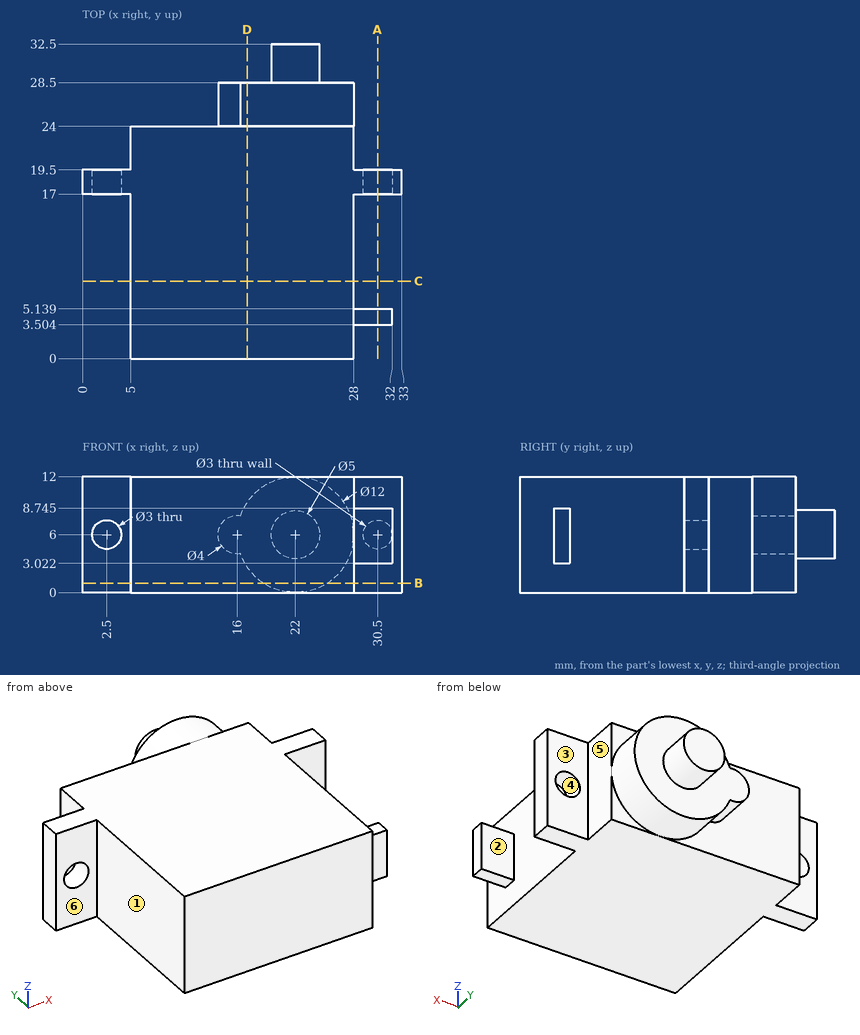
Answer from the drawing. Dimensions are ordinates in mm from the lowest x, y and z of the part. A direction names the side the tool comes from. Coordinates: 2 decimals unless noted, no trailing zeros. Write each loop counter-clockwise with the first axis right and the second up, starting at its lowest first coordinate (ties: lowest second). Pieces come first, ordered by that corner, then holes. Notation, with made-up numbers: M -36.75,76.5 L -28.75,76.5 A7 cw -28.75,85.5 Z; hole C -30,16.25 d11. An arc over 180 degrees is marked long. Put each result on its own line as item: value. Start each with the question number.
1. Which of the six approach directions +Z, -Z, +X, -X, +Y, -Y give full straight-line access (tool end or side, diameter ignored) to the marked faces 1, 2 and 3?
2. A cutting plane is placed at B-B on z = 1. Write down the section's boundary in (x, y).
3. A cutting plane is placed at C-C on y = 8. Write down the section's boundary in (x, z).
4. Flat-ended cylindrical pins translate along their axes: P1, Ø2.5, axis at x = 3, z = 6, coming from the +Y side; P2, Ø2, axis at y = 4.5, z = 2, coming from the -X side; P3, Ø1.8, axis at x = 29.5, y = 4.5, coming from the +Z side (1 decimal). Find the tip coordinate at first contact, or state that the pin passes through.
5. For a pull along X with two mould halves and no side action, classify the marked faces 4, 5 and 6 as pulls with the +X half, pulls with the -X half, needs draft (parallel to the pull), parting line crosses it, or undercut.
6. A cutting plane is placed at A-A on x = 30.5. Write down the section's boundary in (y, z) (1 decimal).
7. A cutting plane is placed at D-D on x = 17. Write down the section's boundary in (y, z).
8. Consider line 1 (X direction, y = 19.05, z = 6); line 2 (Y direction, x = 30.5, z = 4) (1 decimal); line 3 (Z direction, x = 2.5, y = 17.9). Determine where each line is inside the solid, lowest interval first. Write a range as from..to.
Resolved:
1. face 1: +Z, -Z, -X, -Y
1. face 2: +Z, -Z, +X
1. face 3: +Z, -Z, +X, +Y
2. outline: M 0,17 L 5,17 L 5,0 L 28,0 L 28,17 L 33,17 L 33,19.5 L 28,19.5 L 28,24 L 25.32,24 L 25.32,28.5 L 18.68,28.5 L 18.68,24 L 5,24 L 5,19.5 L 0,19.5 Z
3. outline: M 5,0 L 28,0 L 28,12 L 5,12 Z
4. P1: stops at y = 19.5
4. P2: stops at x = 5
4. P3: stops at z = 8.7
5. face 4: undercut
5. face 5: pulls with the +X half
5. face 6: needs draft
6. outline: M 3.5,3 L 5.1,3 L 5.1,8.7 L 3.5,8.7 Z; M 17,0 L 19.5,0 L 19.5,4.5 L 17,4.5 Z; M 17,7.5 L 19.5,7.5 L 19.5,12 L 17,12 Z
7. outline: M 0,0 L 24,0 L 24,2.68 L 28.5,2.68 L 28.5,9.32 L 24,9.32 L 24,12 L 0,12 Z
8. line 1: x = 0..1, 4..29, 32..33
8. line 2: y = 3.5..5.1, 17..19.5
8. line 3: z = 0..4.5, 7.5..12
